Check sheet for the modelled part. Datum: model origin and axes. Units: mm. Face numbers are marked on the shaded views. A direction names the side the tool comes from. Give positions to 0.01 mm unless a question says otherwise; leave off trailing zeros. Order: outer loops, then holes, each group sorted by start corner. A loop starts at its lowest first (then second) coordinate and runs counter-clockwise, first axis right, second up.
```python
from build123d import *

# Parameters (mm, degrees)
BOSS_EXTRUDE1_DEPTH                                 = 31.5
SKETCH2_R                                           = 12
SKETCH2_R_2                                         = 1.65
CUT_EXTRUDE1_DEPTH                                  = 77.591448609
SKETCH3_W                                           = 40
SKETCH3_H                                           = 31
CUT_EXTRUDE2_DEPTH                                  = 81.257398413
BOSS_EXTRUDE2_DEPTH                                 = 5
SKETCH8_W                                           = 68
SKETCH8_H                                           = 8
SKETCH8_W_2                                         = 28
BOSS_EXTRUDE3_DEPTH                                 = 0.6
CBORE_FOR_M4_HEX_SOCKET_HEAD_CAP_SCREW1_D           = 4.5
CBORE_FOR_M4_HEX_SOCKET_HEAD_CAP_SCREW1_CBORE_D     = 10
CBORE_FOR_M4_HEX_SOCKET_HEAD_CAP_SCREW1_CBORE_DEPTH = 8
CHAMFER1_SIZE                                       = 12
CHAMFER2_SIZE                                       = 5


with BuildPart() as part:
    # Sketch1 → Boss-Extrude1 (new, symmetric)
    with BuildSketch(Plane(origin=(0, 0, 0), x_dir=(0, 0, -1), z_dir=(1, 0, 0))):
        Polygon((-55, 0), (0, 0), (0, 12), (-60, 12), (-60, -43), (-55, -43), align=None)
    extrude(amount=BOSS_EXTRUDE1_DEPTH, both=True)

    # Sketch2 → Cut-Extrude1 (cut, through all)
    with BuildSketch(Plane(origin=(0, 0, 55), x_dir=(-1, 0, 0), z_dir=(0, 0, -1))):
        with Locations(Location((0, -22, 0), (0, 0, 90))):
            Circle(SKETCH2_R)
        with Locations(Location((-15.5, -6.5, 0), (0, 0, 90))):
            Circle(SKETCH2_R_2)
        with Locations(Location((-15.5, -37.5, 0), (0, 0, 90))):
            Circle(SKETCH2_R_2)
        with Locations(Location((15.5, -37.5, 0), (0, 0, 90))):
            Circle(SKETCH2_R_2)
        with Locations(Location((15.5, -6.5, 0), (0, 0, 90))):
            Circle(SKETCH2_R_2)
    extrude(amount=-CUT_EXTRUDE1_DEPTH, mode=Mode.SUBTRACT)

    # Sketch3 → Cut-Extrude2 (cut, through all)
    with BuildSketch(Plane.XZ):
        with Locations((-11.5, 15.5)):
            Rectangle(SKETCH3_W, SKETCH3_H)
    extrude(amount=-CUT_EXTRUDE2_DEPTH, mode=Mode.SUBTRACT)

    # Sketch7 → Boss-Extrude2 (add)
    with BuildSketch(Plane(origin=(31.5, 0, 0), x_dir=(0, 0, -1), z_dir=(1, 0, 0))):
        Polygon((-60, -43), (-45, -43), (0, -13), (0, 12), (-60, 12), align=None)
    extrude(amount=BOSS_EXTRUDE2_DEPTH)

    # Sketch8 → Boss-Extrude3 (add)
    with BuildSketch(Plane(origin=(0, 12, 0), x_dir=(1, 0, 0), z_dir=(0, 1, 0))):
        with Locations((2.5, -45)):
            Rectangle(SKETCH8_W, SKETCH8_H)
        with Locations((22.5, -15)):
            Rectangle(SKETCH8_W_2, SKETCH8_H)
    extrude(amount=BOSS_EXTRUDE3_DEPTH)

    # CBORE for M4 Hex Socket Head Cap Screw1 (through all)
    with Locations(Plane(origin=(0, 0, 0), x_dir=(-1, 0, 0), z_dir=(0, -1, 0))):
        with Locations((24.5, -45), (-24.5, -45), (-24.5, -15)):
            CounterBoreHole(CBORE_FOR_M4_HEX_SOCKET_HEAD_CAP_SCREW1_D / 2, CBORE_FOR_M4_HEX_SOCKET_HEAD_CAP_SCREW1_CBORE_D / 2, CBORE_FOR_M4_HEX_SOCKET_HEAD_CAP_SCREW1_CBORE_DEPTH)

    # Chamfer1
    chamfer1_edges = [part.edges().sort_by_distance(p)[0] for p in [
        (-31.5, -43, 57.5),
    ]]
    chamfer(chamfer1_edges, length=CHAMFER1_SIZE)

    # Chamfer2
    chamfer2_edges = [part.edges().sort_by_distance(p)[0] for p in [
        (-31.5, 6, 31),
        (8.5, 6, 0),
    ]]
    chamfer(chamfer2_edges, length=CHAMFER2_SIZE)


solid = part.part
```
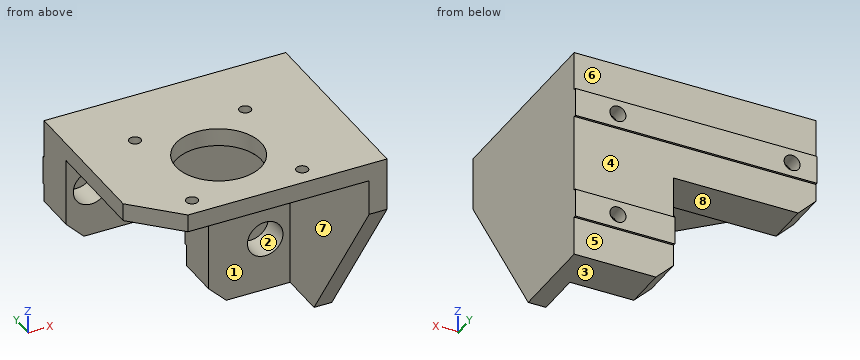
Q1. Material ranges on line 1 (X direction, y = 11.2, z = 45); line 2 (Z direction, x = 24.5, y = 5.5); line 3 (Z direction, x = -24.5, y = 6), recorded low to high.
Q2. Sectioned sample at A-A, the plane z = 15. Record the cut outline in (x, y).
Q3. Go/stop test with flat-tipped pins: P1, Ø5.5, axis at x = 15.5, z = 55, coming from the +Y side; P2, Ø10, axis at x = 13.5, z = 12, coming from the -Y side; P3, Ø6, axis at x = 24.5, z = 15, coming from the -Y side; P4, Ø5, axis at y = -5, z = 53, coming from the -X side. Record where each tip stops, or that it passes through.
Q4. Sectioned sample at D-D, the plane z = 56.5. Record the cut outline in (x, y).
Q5. Tool access check on the marked faces 5, 6, 7 and 8. Record the directions out of +Z, -Z, +X, -X, +Y, -Y that give a thin tool (end or side, any length) a straight path to the whole face; none if there is none.
Q6. Draft check along Z on the marked faces 1, 2, 3 and 4. Enter one of: pulls with the +Z half, pulls with the -Z half, needs draft (parallel to the pull), parting line crosses it, or undercut.
Q7. Sectioned sample at C-C, the plane x = 15.5. Record the cut outline in (y, z), plus the area to 3 significant figures.
Q8. Sectioned sample at B-B, the plane y = -37.5. Record the cut outline in (x, z).
Filled in:
1. line 1: x = -31.5 to -26.75, -22.25 to 22.25, 26.75 to 36.5
1. line 2: z = 0 to 10, 20 to 40, 50 to 60
1. line 3: z = 31 to 40, 50 to 60
2. outline: (8.5, 0) - (19.5, 0) - (19.5, 8) - (22.25, 8) - (22.25, 12.6) - (8.5, 12.6) - close; (26.75, 8) - (29.5, 8) - (29.5, 0) - (31.5, 0) - (31.5, -23) - (36.5, -23) - (36.5, 12.6) - (26.75, 12.6) - close
3. P1: stops at y = 12
3. P2: stops at y = 0
3. P3: stops at y = 8
3. P4: stops at x = -31.5
4. outline: (-31.5, -31) - (-19.5, -43) - (36.5, -43) - (36.5, 12) - (-31.5, 12) - close; hole circle Ø3.3 at (-15.5, -37.5); hole circle Ø3.3 at (-15.5, -6.5); hole circle Ø24 at (0, -22); hole circle Ø3.3 at (15.5, -37.5); hole circle Ø3.3 at (15.5, -6.5)
5. face 5: -Z, +X, -X, +Y
5. face 6: +Z, +X, -X, +Y
5. face 7: -Z, -X, -Y
5. face 8: -Z, -X, +Y, -Y
6. face 1: needs draft
6. face 2: undercut
6. face 3: pulls with the -Z half
6. face 4: undercut
7. outline: (-43, 55) - (-39.15, 55) - (-39.15, 60) - (-43, 60) - close; (-35.85, 55) - (-8.15, 55) - (-8.15, 60) - (-35.85, 60) - close; (-4.85, 55) - (0, 55) - (0, 0) - (12, 0) - (12, 11) - (12.6, 11) - (12.6, 19) - (12, 19) - (12, 41) - (12.6, 41) - (12.6, 49) - (12, 49) - (12, 60) - (-4.85, 60) - close
7. area: 912 mm2
8. outline: (-25, 55) - (-17.15, 55) - (-17.15, 60) - (-25, 60) - close; (-13.85, 55) - (13.85, 55) - (13.85, 60) - (-13.85, 60) - close; (17.15, 55) - (31.5, 55) - (31.5, 36.75) - (36.5, 36.75) - (36.5, 60) - (17.15, 60) - close
